Autodesk Inventor part; units mm, degrees
ref_plane "YZ Plane" through (0, 0, 0) normal (1, 0, 0) x (0, 1, 0)
ref_plane "XZ Plane" through (0, 0, 0) normal (0, 1, 0) x (-1, 0, 0)
ref_plane "XY Plane" through (0, 0, 0) normal (0, 0, 1) x (1, 0, 0)
sketch "Sketch2" plane through (0, 0, 0) normal (0, 0, 1) x (1, 0, 0)
  line L0 (27.933, -48.3814) -> (-27.933, -48.3814)
  line L1 (-27.933, -48.3814) -> (-55.866, 0)
  line L2 (-55.866, 0) -> (-27.933, 48.3814)
  line L3 (-27.933, 48.3814) -> (27.933, 48.3814)
  line L4 (27.933, 48.3814) -> (55.866, 0)
  line L5 (55.866, 0) -> (27.933, -48.3814)
  line L6 (-28.5104, 49.3814) -> (-57.0207, 0)
  line L7 (-57.0207, 0) -> (-28.5104, -49.3814)
  line L8 (-28.5104, -49.3814) -> (28.5104, -49.3814)
  line L9 (28.5104, -49.3814) -> (57.0207, 0)
  line L10 (57.0207, 0) -> (28.5104, 49.3814)
  line L11 (28.5104, 49.3814) -> (-28.5104, 49.3814)
  line L12 (0, -48.3814) -> (0, 48.3814) construction
  line L13 (-55, -1.5) -> (-35.866, -1.5)
  line L14 (-35.866, -1.5) -> (-35.866, -3.4)
  line L15 (-35.866, -3.4) -> (-53.903, -3.4)
  line L16 (55, -1.5) -> (35.866, -1.5)
  line L17 (35.866, -1.5) -> (35.866, -3.4)
  line L18 (35.866, -3.4) -> (53.903, -3.4)
  point P0 (0, 0)
  point P1 (0, 0)
  point P2 (53.903, -3.4)
  point P3 (55, -1.5)
  dimension "d10" = 1
  dimension "d13" = 1.9
  dimension "d14" = 20
  dimension "d15" = 1.5
  dimension "d28" = 110
extrude "Extrusion2" add sketch "Sketch2" along normal mid plane 1.5 contours L0 L1 L15 L14 L13 L2 L3 L4 L5 L16 L17 L18 | L11 L10 L9 L8 L7 L6
sketch "Sketch5" plane through (0, 0, 0) normal (0, 1, 0) x (-1, 0, 0)
  line L0 (0, 0) -> (-10.6377, 0)
  line L1 (-10.6377, 0) -> (-7.4876, 0)
  line L2 (0, 0) -> (0, 10)
  arc A0 (10.6377, 0) -> (-10.6377, 0) centre (0, 10) ccw
  line L3 (0, 0) -> (10.6377, 0)
  line L4 (28.5104, 0.75) -> (-28.5104, 0.75)
  line L5 (0, 0.75) -> (0, 24.6)
  point P0 (-11.2959, 0.75)
  point P1 (0, 0.75)
  dimension "d29" = 10
  dimension "d30" = 14.6
revolve "Revolution3" add sketch "Sketch5" angle 360 about axis through (0, 0, 0.75) along (0, 0, 1) picked at (-3.7653, 3.8333) contours L4 A0 L5 L2
fillet "Fillet2" radius 5 1 edges at (-11.2959, 0, 0.75)
properties part number "CUERPO_ABEJA"
The listing builds one solid part. Answer for the finished solid, in the listing's coordinates (mm). Give positions to 0.01 mm unless a question says otherwise; leave off trailing zeros. Loops run counter-clockwise (first coordinate to the right, second up) from the corner with the lowest first, then second, coordinate; pieces in that order, holes last. Notation, with made-up numbers: (25.5, -35) - (68.5, -35) arc R22 ccw to (68.5, -25) - close; hole circle Ø2 at (76.5, 12). An arc over 180 degrees is marked (long way). Answer as a JSON object with one key per item and string values.
1. Flat-ended cylindrical pins translate along their axes: pin 1 Ø1.6 at (x, z) = (45, 0.5) entering from +Y; pin 2 Ø0.8 at (y, z) = (-2, -0.5) entering from -X; pin 3 Ø1.6 at (x, z) = (-47, 0.5) entering from +Y. Find the tip coordinate at first contact, or state that the pin passes through.
Determined:
{"pin 1": "y = 22.21", "pin 2": "x = -56.1", "pin 3": "y = 18.74"}
2. Find the intervals of material crossed by L1, parallel to Z at x = -13.5, y = -20.5; L2, parallel to Z at x = -12, y = 12.5; L3, parallel to Y at x = 0.5, z = 7, in increasing order. Write a range as [from, to].
Determined:
{"L1": "[-0.75, 0.75]", "L2": "[-0.75, 1.09]", "L3": "[-14.28, 14.28]"}
3. A cutting plane is placed at C-C (y = -20.5). Write down the section's boundary in (x, z), then the cut area to 3 significant figures.
Determined:
{"outline": "(-45.19, -0.75) - (45.19, -0.75) - (45.19, 0.75) - (-45.19, 0.75) - close", "area": "136 mm²"}
4. For a pull along X with two mould halves and no side action, classify faces 1 (the flat face through (25, 1, 0.75)), 2 (the flat face through (42.566, -25.036, -0.01)), 3 (the flat face through (-42.566, 25.036, -0.01)) as pulls with the +X half, pulls with the -X half, needs draft (parallel to the pull), parting line crosses it, or undercut.
Determined:
{"face 1": "needs draft", "face 2": "pulls with the +X half", "face 3": "pulls with the -X half"}
5. A cutting plane is placed at D-D (z = 22.25). Write down the section's boundary in (x, y), then the cut area to 3 significant figures.
Determined:
{"outline": "circle Ø15.89 at (0, 0)", "area": "198 mm²"}
6. A cutting plane is placed at B-B (x = -42). Write down the section's boundary in (y, z), then the cut area to 3 significant figures.
Determined:
{"outline": "(-26.02, -0.75) - (-3.4, -0.75) - (-3.4, 0.75) - (-26.02, 0.75) - close; (-1.5, -0.75) - (26.02, -0.75) - (26.02, 0.75) - (-1.5, 0.75) - close", "area": "75.2 mm²"}
7. A cutting plane is placed at A-A (x = 44). Write down the section's boundary in (y, z).
Determined:
{"outline": "(-22.55, -0.75) - (-3.4, -0.75) - (-3.4, 0.75) - (-22.55, 0.75) - close; (-1.5, -0.75) - (22.55, -0.75) - (22.55, 0.75) - (-1.5, 0.75) - close"}
